```python
from build123d import *

# Parameters (mm, degrees)
ESQUISSE1_W        = 62
ESQUISSE1_H        = 37
BOSS_EXTRU_1_DEPTH = 28
COQUE1_T           = -1
CONG_1_R           = 1
ESQUISSE2_W        = 1
ESQUISSE2_H        = 25
BOSS_EXTRU_2_DEPTH = 1
CONG_2_R           = 1


with BuildPart() as part:
    # Esquisse1 → Boss.-Extru.1 (new body)
    with BuildSketch(Plane.XY):
        with Locations((31, 18.5)):
            Rectangle(ESQUISSE1_W, ESQUISSE1_H)
    extrude(amount=BOSS_EXTRU_1_DEPTH)

    # Coque1
    coque1_openings = [part.faces().sort_by_distance(p)[0] for p in [
        (31, 18.5, 28),
    ]]
    offset(amount=COQUE1_T, openings=coque1_openings, kind=Kind.INTERSECTION)

    # Congé1
    cong_1_edges = [part.edges().sort_by_distance(p)[0] for p in [
        (1, 18.5, 1),
        (1, 36, 14.5),
        (31, 1, 1),
        (1, 1, 14.5),
        (61, 18.5, 1),
        (61, 1, 14.5),
        (31, 36, 1),
        (61, 36, 14.5),
        (1, 18.5, 28),
        (31, 1, 28),
        (61, 18.5, 28),
        (31, 36, 28),
    ]]
    fillet(cong_1_edges, radius=CONG_1_R - 0.0001)  # a hair under: the kernel refuses the full size

    # Esquisse2 → Boss.-Extru.2 (add)
    with BuildSketch(Plane.XY.offset(1)):
        with Locations((15, 18.5)):
            Rectangle(ESQUISSE2_W, ESQUISSE2_H)
        with Locations((46, 18.5)):
            Rectangle(ESQUISSE2_W, ESQUISSE2_H)
    extrude(amount=BOSS_EXTRU_2_DEPTH)

    # Congé2
    cong_2_edges = [part.edges().sort_by_distance(p)[0] for p in [
        (46, 31, 1),
        (15, 31, 1),
        (46, 6, 1),
        (15, 6, 1),
        (46.5, 18.5, 1),
        (15.5, 18.5, 1),
        (45.5, 18.5, 1),
        (14.5, 18.5, 1),
    ]]
    fillet(cong_2_edges, radius=CONG_2_R - 0.0001)  # a hair under: the kernel refuses the full size


solid = part.part
```
Verification items for the finished model (mm, model axes). A direction names the side the tool comes from. Coordinates: 2 decimals unless noted, no trailing zeros. Order: outer loops, then holes, each group sorted by start corner. A loop starts at its lowest first (then second) coordinate and runs counter-clockwise, first axis right, second up. Notation, with made-up numbers: (-31.5, 1.5) -> (21.5, 1.5) arc R13 ccw to (21.5, 7.5) -> close; hole circle Ø6 at (55.25, -1.75). An arc over 180 degrees is marked (long way). Answer as CSV lines item,"result". Start each with the question number.
1) Release check for a two-part mould opening along X. For faces 1 (the face through (31, 19, 0)), 2 (the face through (62, 18, 14)), 3 (the face through (31, 1, 14)) record: released by +X, released by -X, zero draft, split by the parting line, or undercut.
2) Material ranges on L1, parallel to Y at x = 38, z = 5.5; L2, parallel to X at y = 35, z = 12.25; L3, parallel to Z at x = 21, y = 10.5, recorded low to high. Write a range as [from, to].
3) Gauge pin test, flat ends, axial feed: pin 1 Ø16.5 at (x, y) = (32.5, 22) entering from +Z; pin 2 Ø1 at (x, z) = (29, 6) entering from -Y; pin 3 Ø1.1 at (x, y) = (46, 20) entering from +Z; pin 4 Ø6 at (x, y) = (26, 4.5) entering from +Z. Record the tip position at first contact, or that the pin passes through.
4) Set-up check for faces 4 (the face through (1, 18, 14)), 5 (the face through (31, 0, 14)): record each of +Z, -Z, +X, -X, +Y, -Y from which the full face is reachable in a straight line by a thin tool's end or side.
5) Cross-section at A-A, the plane z = 6.75. Record the boundary of the cut face in (x, y).
Conclusion:
1,face 1,"zero draft"
1,face 2,"released by +X"
1,face 3,"undercut"
2,L1,"y = [0, 1], [36, 37]"
2,L2,"x = [0, 1], [61, 62]"
2,L3,"z = [0, 1]"
3,pin 1,"stops at z = 1"
3,pin 2,"stops at y = 0"
3,pin 3,"stops at z = 2"
3,pin 4,"stops at z = 1.13"
4,face 4,"+Z"
4,face 5,"+Z, -Z, +X, -X, -Y"
5,outline,"(0, 0) -> (62, 0) -> (62, 37) -> (0, 37) -> close; hole (1, 2) arc R1 ccw to (2, 1) -> (60, 1) arc R1 ccw to (61, 2) -> (61, 35) arc R1 ccw to (60, 36) -> (2, 36) arc R1 ccw to (1, 35) -> close"
